For this review, use the dimensioned drawing (mm, ordinates from the lowest corner) and the shaded views. A direction names the side the tool comes from. Give positions to 0.01 mm unless a question says otherwise; leave off trailing zeros. Loops run counter-clockwise (first coordinate to the right, second up) from the corner with the lowest first, then second, coordinate; pieces in that order, holes last. Notation, with made-up numbers: M 38.5,47.5 L 61.5,47.5 A12 cw 61.5,61.5 Z; hole C 2.25,86 d11. An arc over 180 degrees is marked long. Use a Markdown table: item, result. Add a question column.
(1) For probe 1 along Y at (x, z) = (97, 16); probe 2 along X at (y, z) = (21.25, 36.5); probe 3 along Y at (x, z) = (54, 41.5), list the stretches that pass through material, from the lowest coordinate up.
(2) Add section B-B, the plane z = 36.5. Give the boundary of the cut face in (x, y), then the cut area to 3 significant figures.
(3) For the marked faces 1, 2 and 3, list the 3-axis set-ups (+Z, -Z, +X, -X, +Y, -Y) from which the entire face can be reached by the end or side of a thin tool; tool diameter is ignored.
(4) Insertion check: pin 1 Ø5 at (x, y) = (97, 10) entering from +Z; pin 2 Ø5 at (y, z) = (12, 7.5) entering from +X; pin 3 Ø3 at (y, z) = (14.5, 25) entering from -X. Each pin has a flat end and moves straight along its axis. Give the tip position at first contact, or say it passes through.
(5) Add section C-C, the plane x = 97. Give the boundary of the cut face in (y, z), then the cut area to 3 significant figures.
(6) Add section D-D, the plane y = 8. Give the boundary of the cut face in (x, z).
(7) Add section A-A, the plane x = 4.1. Give the boundary of the cut face in (y, z), then the cut area to 3 significant figures.
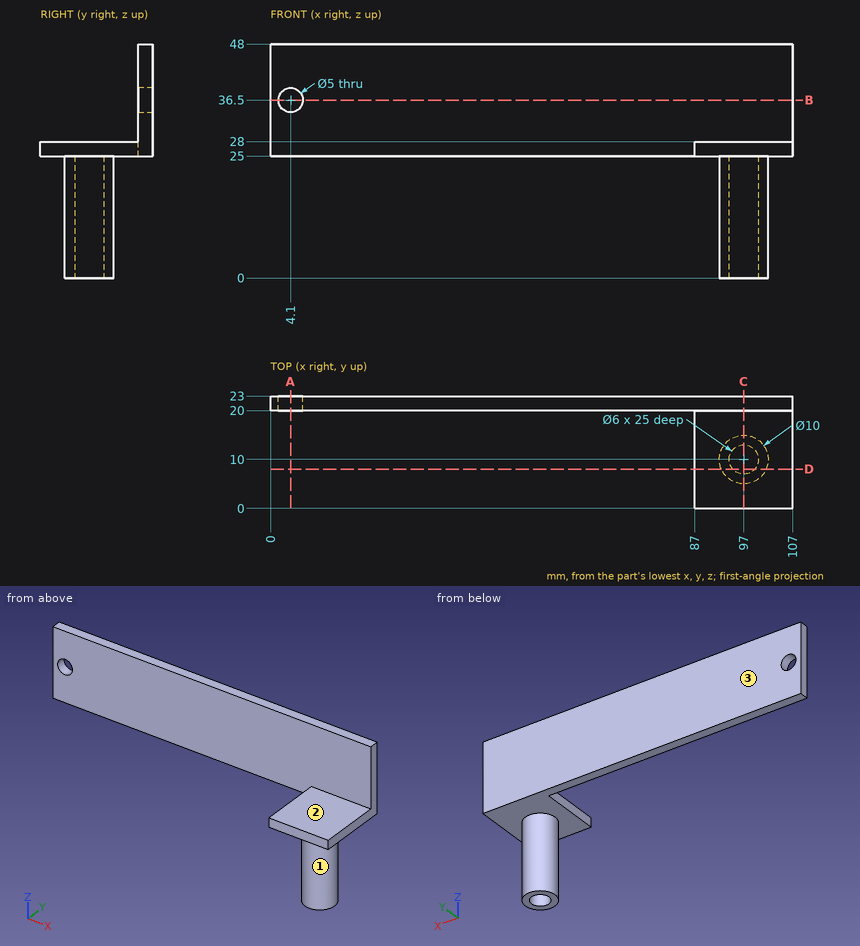
Established:
| question | item | result |
|---|---|---|
| 1 | probe 1 | 5 to 7, 13 to 15 |
| 1 | probe 2 | 0 to 1.6, 6.6 to 107 |
| 1 | probe 3 | 20 to 23 |
| 2 | outline | M 0,20 L 1.6,20 L 1.6,23 L 0,23 Z; M 6.6,20 L 107,20 L 107,23 L 6.6,23 Z |
| 2 | area | 306 mm^2 |
| 3 | face 1 | -Z |
| 3 | face 2 | +Z, +X, -X, -Y |
| 3 | face 3 | +Z, -Z, +X, -X, +Y |
| 4 | pin 1 | z = 28 |
| 4 | pin 2 | x = 102 |
| 4 | pin 3 | x = 87 |
| 5 | outline | M 0,25 L 5,25 L 5,0 L 7,0 L 7,25 L 13,25 L 13,0 L 15,0 L 15,25 L 23,25 L 23,48 L 20,48 L 20,28 L 0,28 Z |
| 5 | area | 229 mm^2 |
| 6 | outline | M 87,25 L 92.42,25 L 92.42,0 L 94.76,0 L 94.76,25 L 99.24,25 L 99.24,0 L 101.58,0 L 101.58,25 L 107,25 L 107,28 L 87,28 Z |
| 7 | outline | M 20,25 L 23,25 L 23,34 L 20,34 Z; M 20,39 L 23,39 L 23,48 L 20,48 Z |
| 7 | area | 54.0 mm^2 |
